Design review of the part built by this model. Coordinates are the model's own, in mm. Coordinates: 2 decimals unless noted, no trailing zeros. Loops run counter-clockwise (first coordinate to the right, second up) from the corner with the lowest first, then second, coordinate; pieces in that order, holes last. Notation, with made-up numbers: (-24, 57.25) -> (-7, 57.25) arc R12 ccw to (-7, 77.25) -> close; hole circle Ø11 at (56, 66). An arc over 180 degrees is marked (long way). Answer as a JSON object with one key per item and string values.
```python
from build123d import *

# Parameters (mm, degrees)
F0_W     = 110
F0_H     = 100
F1_DEPTH = 10
F2_R     = 2
F3_DEPTH = 25
F4_W     = 110
F4_H     = 100
F5_DEPTH = 10


with BuildPart() as f1:
    # F0 (on Front) → F1 (new body)
    with BuildSketch(Plane.XZ):
        Rectangle(F0_W, F0_H)
    extrude(amount=F1_DEPTH)

    # F2 (on face) → F3 (cut)
    with BuildSketch(Plane.XZ.offset(10)):
        with Locations((-46, 41)):
            Circle(F2_R)
        with Locations((-20, 41)):
            Circle(F2_R)
        with Locations((-46, 19)):
            Circle(F2_R)
        with Locations((-20, 19)):
            Circle(F2_R)
        with Locations((46, 41)):
            Circle(F2_R)
        with Locations((20, 41)):
            Circle(F2_R)
        with Locations((20, 19)):
            Circle(F2_R)
        with Locations((46, 19)):
            Circle(F2_R)
        with Locations((-46, -19)):
            Circle(F2_R)
        with Locations((-46, -41)):
            Circle(F2_R)
        with Locations((-20, -19)):
            Circle(F2_R)
        with Locations((-20, -41)):
            Circle(F2_R)
        with Locations((20, -41)):
            Circle(F2_R)
        with Locations((46, -41)):
            Circle(F2_R)
        with Locations((46, -19)):
            Circle(F2_R)
        with Locations((20, -19)):
            Circle(F2_R)
    extrude(amount=-F3_DEPTH, mode=Mode.SUBTRACT)

    # F4 (on Front) → F5 (join)
    with BuildSketch(Plane.XZ):
        with Locations((0, -100)):
            Rectangle(F4_W, F4_H)
    extrude(amount=F5_DEPTH)


solid = f1.part
```
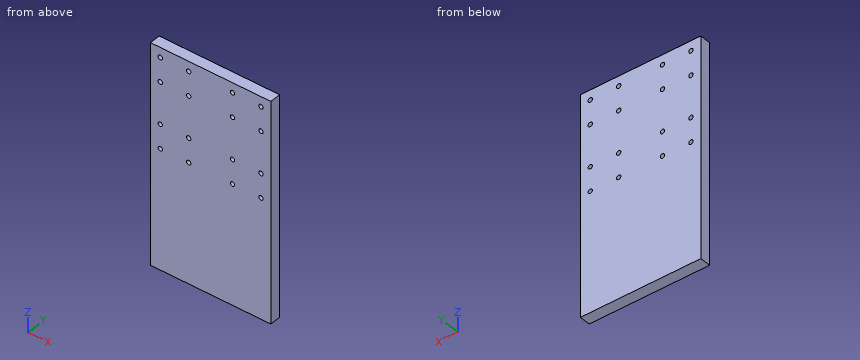
1) Add section B-B, the plane z = -19. Give the boundary of the cut face in (x, y), and give its area (3 significant figures).
Completed:
{"outline": "(-55, -10) -> (-48, -10) -> (-48, 0) -> (-55, 0) -> close; (-44, -10) -> (-22, -10) -> (-22, 0) -> (-44, 0) -> close; (-18, -10) -> (18, -10) -> (18, 0) -> (-18, 0) -> close; (22, -10) -> (44, -10) -> (44, 0) -> (22, 0) -> close; (48, -10) -> (55, -10) -> (55, 0) -> (48, 0) -> close", "area": "940 mm²"}
2) Wall thickness on probe 1 along Z at (x, y) = (-20, -2.25); probe 2 along X at (y, z) = (-3.75, -39.5): over which ranges is each line inside the solid? List them lowest first.
Completed:
{"probe 1": "-150 to -43, -39 to -21, -17 to 17, 21 to 39, 43 to 50", "probe 2": "-55 to -47.32, -44.68 to -21.32, -18.68 to 18.68, 21.32 to 44.68, 47.32 to 55"}
3) Add section A-A, the plane x = -46. Give the boundary of the cut face in (y, z).
Completed:
{"outline": "(-10, -150) -> (0, -150) -> (0, -43) -> (-10, -43) -> close; (-10, -39) -> (0, -39) -> (0, -21) -> (-10, -21) -> close; (-10, -17) -> (0, -17) -> (0, 17) -> (-10, 17) -> close; (-10, 21) -> (0, 21) -> (0, 39) -> (-10, 39) -> close; (-10, 43) -> (0, 43) -> (0, 50) -> (-10, 50) -> close"}
